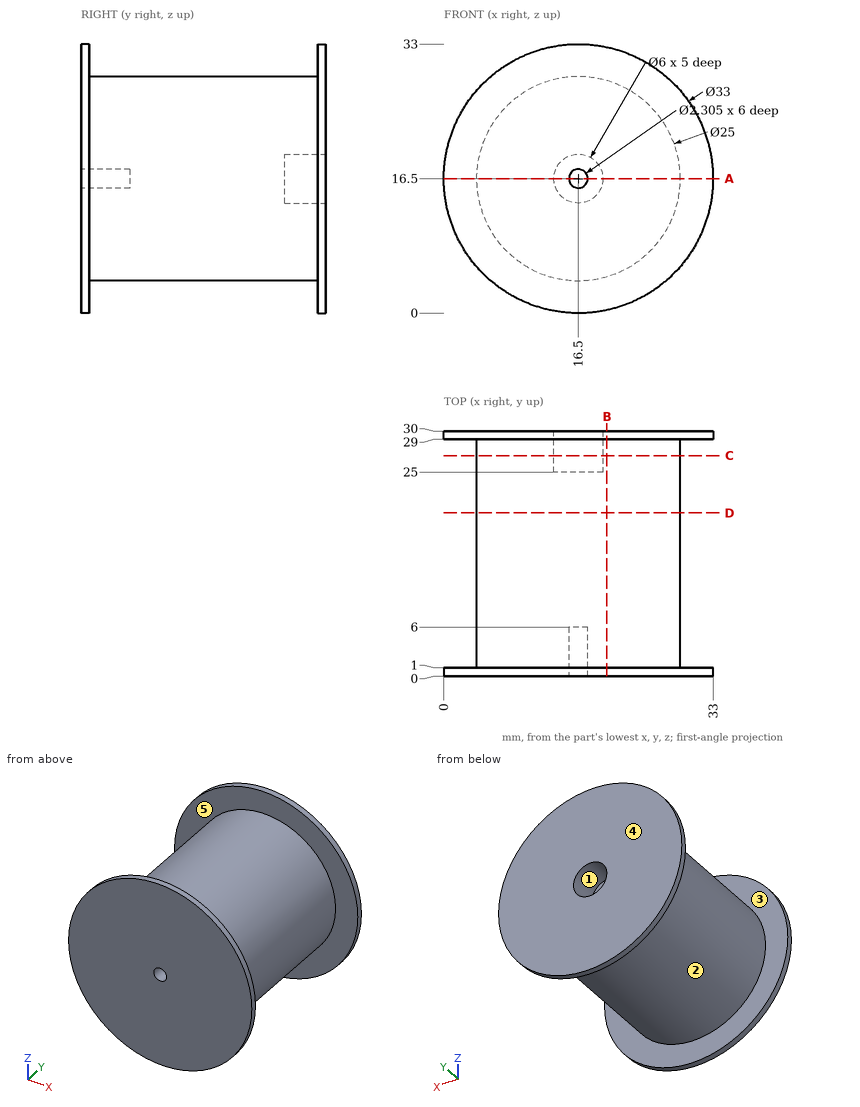
Geometry: see drawing. Coordinates: mm, zero at the bounding-box minimum. A direction names the side the tool comes from. Coordinates: 2 decimals unless noted, no trailing zeros. Order: outer loops, then holes, each group sorted by start corner. A loop starts at its lowest first (then second) coordinate and runs counter-clockwise, first axis right, second up. Notation, with made-up numbers: (15, -11) - (46, -11) arc R14 ccw to (46, 9) - close; hole circle Ø8 at (-36.5, -5.5). An arc over 180 degrees is marked (long way). Write each question's results on one line, items separated by ' | '.
1) Set-up query: the marked faces 4 and 5. Return all of +Z, -Z, +X, -X, +Y, -Y with unobstructed straight access to the full face (end or side cutting, diameter ignored); none if empty.
Results list:
face 4: +Z, -Z, +X, -X, +Y | face 5: none
2) Section B-B, the plane x = 20. Return loops of the section in (y, z).
Results list:
outline: (0, 0.38) - (1, 0.38) - (1, 4.5) - (29, 4.5) - (29, 0.38) - (30, 0.38) - (30, 32.62) - (29, 32.62) - (29, 28.5) - (1, 28.5) - (1, 32.62) - (0, 32.62) - close
3) Pin query (flat end, axial travel): pin 1 (3 mm diameter, centred on x = 29.5, y = 16.5, fed in from +Z); pin 2 (1.5 mm diameter, centred on y = 6.5, z = 26.5, fed in from -X); pin 3 (5 mm diameter, centred on x = 16.5, z = 16.5, fed in from +Y); pin 4 (10 mm diameter, centred on x = 20.5, z = 11, fed in from -Y). Return the tip coordinate at first contact, or that it passes through.
Results list:
pin 1: z = 21.4 | pin 2: x = 8.09 | pin 3: y = 25 | pin 4: y = 0
4) Section D-D, the plane y = 20. Return loops of the section in (x, z).
Results list:
outline: circle Ø25 at (16.5, 16.5)
5) Pull-direction query (X, two-part tool) for the marked faces 1, 2 and 3; classes: pulls with the +X half, pulls with the -X half, needs draft (parallel to the pull), parting line crosses it, or undercut.
Results list:
face 1: undercut | face 2: parting line crosses it | face 3: needs draft
6) Section A-A, the plane z = 16.5. Return loops of the section in (x, y), plus the area to 3 significant figures.
Results list:
outline: (0, 0) - (15.35, 0) - (15.35, 6) - (17.65, 6) - (17.65, 0) - (33, 0) - (33, 1) - (29, 1) - (29, 29) - (33, 29) - (33, 30) - (19.5, 30) - (19.5, 25) - (13.5, 25) - (13.5, 30) - (0, 30) - (0, 29) - (4, 29) - (4, 1) - (0, 1) - close | area: 722 mm^2
7) Section C-C, the plane y = 27. Return loops of the section in (x, z), plus the area to 3 significant figures.
Results list:
outline: circle Ø25 at (16.5, 16.5); hole circle Ø6 at (16.5, 16.5) | area: 463 mm^2
8) Line query: line 1 (Z direction, x = 16.5, y = 28.1); line 2 (Y direction, x = 5, z = 26.5); line 3 (Z direction, x = 16.5, y = 3.5). Output: solid intervals per line, ascending. Write a range as from..to.
Results list:
line 1: 4..13.5, 19.5..29 | line 2: 0..1, 29..30 | line 3: 4..15.35, 17.65..29
